```python
from build123d import *

# Parameters (mm, degrees)
SKETCH_R        = 16
PAD_DEPTH       = 20
SKETCH001_R     = 11.2
POCKET_DEPTH    = 20.001
SKETCH002_W     = 8
SKETCH002_H     = 19
PAD001_DEPTH    = 12
POCKET001_DEPTH = 3
SKETCH008_R     = 2.8
POCKET002_DEPTH = 15


with BuildPart() as part:
    # Sketch → Pad (new body)
    with BuildSketch(Plane.XY):
        Circle(SKETCH_R)
    extrude(amount=PAD_DEPTH)

    # Sketch001 → Pocket (cut, through all)
    with BuildSketch(Plane.XY.offset(20)):
        Circle(SKETCH001_R)
    extrude(amount=-POCKET_DEPTH, mode=Mode.SUBTRACT)

    # Sketch002 → Pad001 (new body)
    with BuildSketch(Plane.XY.offset(20)):
        with Locations((17, 0)):
            Rectangle(SKETCH002_W, SKETCH002_H)
    extrude(amount=-PAD001_DEPTH)

    # Sketch005 → Pocket001 (cut, symmetric)
    with BuildSketch(Plane(origin=(13, 0, 0), x_dir=(0, -1, 0), z_dir=(-1, 0, 0))):
        Polygon((0, 9.207993), (4.15, 11.603996), (4.15, 16.396004), (0, 18.792007), (-4.15, 16.396004), (-4.15, 11.603996), align=None)
    extrude(amount=POCKET001_DEPTH, both=True, mode=Mode.SUBTRACT)

    # Sketch008 → Pocket002 (cut)
    with BuildSketch(Plane.YZ.offset(21)):
        with Locations((0, 14)):
            Circle(SKETCH008_R)
    extrude(amount=-POCKET002_DEPTH, mode=Mode.SUBTRACT)


solid = part.part
```
Could you check a few things on this model? Use its own coordinates, in mm. A direction names the side the tool comes from. Coordinates: 2 decimals unless noted, no trailing zeros. Write each loop counter-clockwise with the first axis right and the second up, starting at its lowest first coordinate (ties: lowest second). Pieces come first, ordered by that corner, then holes. Notation, with made-up numbers: (27.25, -25) -> (79.25, -25) arc R28 ccw to (79.25, 3) -> close; hole circle Ø5 at (79.25, -13). An arc over 180 degrees is marked (long way). Write item = value, one per line. Start each with the question number.
(1) I want a section at A-A (x = 0). Please give me the cut outline in (y, z), plus the area to 3 significant figures.
(2) I need wall thicknesses on line 1 (Y direction, x = 0, z = 4); line 2 (Y direction, x = 14, z = 15.25); line 3 (X direction, y = 6, z = 14.75). Which ranges of each line are inside material? Lowest first, please. Write a range as [from, to].
(3) I want a section at C-C (y = 3.5). Please give me the cut outline in (x, z).
(4) Will these pins go through, and if not, where does the flat tip stop? pin 1 (6.5 mm diameter, centred on x = 15.5, y = 0, fed in from -Z); pin 2 (1 mm diameter, centred on y = -5, z = 8.5, fed in from -X); pin 3 (4 mm diameter, centred on x = 18, z = 12.5, fed in from +Y); pin 4 (4 mm diameter, centred on x = 14, z = 13.5, fed in from +Y).
(5) We'd pull the mould along Y, two halves only. Please class faces 4 (the face through (18.535, -0.607, 11.267)), 5 (the face through (18, 0, 8)), 6 (the face through (17, -9.5, 14)): released by +Y, released by -Y, zero draft, split by the parting line, or undercut.
(6) I want a section at B-B (z = 17.25). Please give me the cut outline in (x, y).
(7) I want a section at D-D (z = 14). Please give me the cut outline in (x, y), plus the area to 3 significant figures.
(8) Which directions (+Z, -Z, +X, -X, +Y, -Y) give clear straight access to the entire face, cutting with the end or side of a thin tool? Please do faces 1 (the face through (-11.19, 0.49, 10.14)), 2 (the face through (17, 9.5, 14)), 3 (the face through (13.16, 2.05, 17.61)).
Result set:
q1.outline = (-16, 0) -> (-11.2, 0) -> (-11.2, 20) -> (-16, 20) -> close; (11.2, 0) -> (16, 0) -> (16, 20) -> (11.2, 20) -> close
q1.area = 192 mm2
q2.line_1 = [-16, -11.2], [11.2, 16]
q2.line_2 = [-9.5, -4.15], [4.15, 9.5]
q2.line_3 = [-14.83, -9.46], [9.46, 21]
q3.outline = (-15.61, 0) -> (-10.64, 0) -> (-10.64, 20) -> (-15.61, 20) -> close; (10.64, 0) -> (15.61, 0) -> (15.61, 8) -> (21, 8) -> (21, 20) -> (10.64, 20) -> (10.64, 16.77) -> (16, 16.77) -> (16, 11.23) -> (10.64, 11.23) -> close
q4.pin_1 = 0
q4.pin_2 = -15.35
q4.pin_3 = 9.5
q4.pin_4 = 10.58
q5.face_4 = undercut
q5.face_5 = zero draft
q5.face_6 = released by -Y
q6.outline = (13, -9.5) -> (21, -9.5) -> (21, 9.5) -> (13, 9.5) -> (13, 9.33) arc R16 ccw (long way) to (13, -9.33) -> close; hole (10.88, -2.67) -> (16, -2.67) -> (16, 2.67) -> (10.88, 2.67) arc R11.2 ccw (long way) to start
q7.outline = (10.4, -4.15) arc R11.2 cw (long way) to (10.4, 4.15) -> (16, 4.15) -> (16, 2.8) -> (21, 2.8) -> (21, 9.5) -> (13, 9.5) -> (13, 9.33) arc R16 ccw (long way) to (13, -9.33) -> (13, -9.5) -> (21, -9.5) -> (21, -2.8) -> (16, -2.8) -> (16, -4.15) -> close
q7.area = 454 mm2
q8.face_1 = +Z, -Z
q8.face_2 = +Z, -Z, +X, +Y
q8.face_3 = none
